```python
from build123d import *

# Parameters (mm, degrees)
F1_DEPTH = 3
F3_DEPTH = 25


with BuildPart() as f1:
    # F0 (on Front) → F1 (new body)
    with BuildSketch(Plane.XZ):
        with BuildLine():
            ThreePointArc((50, 21), (49.12132, 23.12132), (47, 24))
            Line((47, 24), (-47, 24))
            ThreePointArc((-47, 24), (-49.12132, 23.12132), (-50, 21))
            Line((-50, 21), (-50, -21))
            ThreePointArc((-50, -21), (-49.12132, -23.12132), (-47, -24))
            Line((-47, -24), (47, -24))
            ThreePointArc((47, -24), (49.12132, -23.12132), (50, -21))
            Line((50, -21), (50, 21))
        make_face()
    extrude(amount=F1_DEPTH)

    # F2 (on face) → F3 (cut)
    with BuildSketch(Plane.XZ.offset(3)):
        with BuildLine():
            Line((30.5, -4.5), (39.5, -4.5))
            ThreePointArc((39.5, -4.5), (44, 0), (39.5, 4.5))
            Line((39.5, 4.5), (30.5, 4.5))
            ThreePointArc((30.5, 4.5), (26, 0), (30.5, -4.5))
        make_face()
        with BuildLine():
            ThreePointArc((-30.5, -4.5), (-26, 0), (-30.5, 4.5))
            Line((-30.5, 4.5), (-39.5, 4.5))
            ThreePointArc((-39.5, 4.5), (-44, 0), (-39.5, -4.5))
            Line((-39.5, -4.5), (-30.5, -4.5))
        make_face()
    extrude(amount=-F3_DEPTH, mode=Mode.SUBTRACT)


solid = f1.part
```
The model under review builds one solid part; all positions refer to its coordinate system, in mm. A direction names the side the tool comes from. Round coordinates to 2 decimals unless told otherwise and drop trailing zeros. Loops run counter-clockwise (first coordinate to the right, second up) from the corner with the lowest first, then second, coordinate; pieces in that order, holes last. Notation, with made-up numbers: (28.25, 2.25) - (70.25, 2.25) arc R36 ccw to (70.25, 40.25) - close; hole circle Ø7 at (-24.75, 1). An arc over 180 degrees is marked (long way). Write each question's results on one line, items separated by ' | '. Start each with the question number.
Q1. Take a section at A-A on z = 0. Give the boundary of the cut face in (x, y), plus the area to 3 significant figures.
Q2. Wall thickness on line 1 along Z through (x, y) = (-38, -1.8); line 2 along X through (y, z) = (-2.55, 1); line 3 along X through (y, z) = (-1.6, 2): over which ranges is each line inside the solid? List them lowest first. Write a range as [from, to].
Q3. Tool access review of faces 1 (the flat face through (-1, -1, -24)), 2 (the cylindrical face through (-26, -2, 0)): name each direction out of +Z, -Z, +X, -X, +Y, -Y from which nothing blocks a thin tool from reaching the whole face with its end or side.
Q4. Take a section at C-C on y = -1.55. Give the boundary of the cut face in (x, z).
Q5. Take a section at B-B on x = 31.5. Give the boundary of the cut face in (y, z).
Q6. Take a section at D-D on x = -43. Give the boundary of the cut face in (y, z), plus the area to 3 significant figures.
Q7. Draft analysis for pull direction Z (two halves, no side actions). For faces 3 (the cylindrical face through (-49.1, -1.48, 23.14)), 4 (the flat face through (35, -2, 4.5)), 5 (the cylindrical face through (49.1, -1.48, -23.14)), state which applies: pulls with the +Z half, pulls with the -Z half, needs draft (parallel to the pull), parting line crosses it, or undercut.
Data:
1) outline: (-50, -3) - (-44, -3) - (-44, 0) - (-50, 0) - close; (-26, -3) - (26, -3) - (26, 0) - (-26, 0) - close; (44, -3) - (50, -3) - (50, 0) - (44, 0) - close | area: 192 mm²
2) line 1: z = [-24, -4.5], [4.5, 24] | line 2: x = [-50, -43.89], [-26.11, 26.11], [43.89, 50] | line 3: x = [-50, -43.53], [-26.47, 26.47], [43.53, 50]
3) face 1: -Z, +X, -X, +Y, -Y | face 2: +Y, -Y
4) outline: (-50, -21) arc R3 ccw to (-47, -24) - (47, -24) arc R3 ccw to (50, -21) - (50, 21) arc R3 ccw to (47, 24) - (-47, 24) arc R3 ccw to (-50, 21) - close; hole (-39.5, -4.5) - (-30.5, -4.5) arc R4.5 ccw to (-30.5, 4.5) - (-39.5, 4.5) arc R4.5 ccw to start; hole (30.5, -4.5) - (39.5, -4.5) arc R4.5 ccw to (39.5, 4.5) - (30.5, 4.5) arc R4.5 ccw to start
5) outline: (-3, -24) - (0, -24) - (0, -4.5) - (-3, -4.5) - close; (-3, 4.5) - (0, 4.5) - (0, 24) - (-3, 24) - close
6) outline: (-3, -24) - (0, -24) - (0, -2.83) - (-3, -2.83) - close; (-3, 2.83) - (0, 2.83) - (0, 24) - (-3, 24) - close | area: 127 mm²
7) face 3: pulls with the +Z half | face 4: undercut | face 5: pulls with the -Z half
